Design review of the part built by this model. Coordinates are the model's own, in mm. Coordinates: 2 decimals unless noted, no trailing zeros. Loops run counter-clockwise (first coordinate to the right, second up) from the corner with the lowest first, then second, coordinate; pieces in that order, holes last. Notation, with made-up numbers: (41.5, 57) -> (72.5, 57) arc R22 ccw to (72.5, 93) -> close; hole circle Ø7 at (50.5, 54.5). An arc over 180 degrees is marked (long way). Use one line per item in the form item = value. Start each with the question number.
1. Consider section B-B (z = -2.5). State how many separate pieces and enclosed holes the cut face has, then the cut area to 3 significant figures.
2. Consider section D-D (y = -86). State the section outline as (x, z) points.
3. Consider section C-C (x = 68). State the section outline as (y, z) points, then the cut area to 3 significant figures.
4. For pin 1 (3 mm diameter, centred on x = 131.76, y = 19.05, fed in from +Z); pin 2 (1.5 mm diameter, centred on x = -48, z = -1, fed in from -Y); pin 3 (1.6 mm diameter, centred on x = 122.5, z = -2.5, fed in from -Y), all flat-tipped, find the tip position at first contact; note any pin that passes through.
5. The part is to be moulded in two halves that separate along X. For faces 1 (the face through (-4.716, -75.824, -1.609)), 2 (the face through (-51.9, -11.8, -1.6)), 3 (the face through (35.69, -25.25, -1.65)), say which applies: released by +X, released by -X, zero draft, split by the parting line, or undercut.
6. Consider section A-A (y = -19.05). State the section outline as (x, z) points, then the cut area to 3 significant figures.
7. Wall thickness on line 1 (Y direction, x = 99, z = -1.95); line 2 (X direction, y = -29.5, z = -0.95): over which ranges is each line inside the solid? List them lowest first. Write a range as from..to.
from build123d import *

# Parameters (mm, degrees)
SKETCH1_W                    = 158.75
SKETCH1_H                    = 63.5
BASE_FLANGE1_DEPTH           = 3.2639
F_10_0_1935_DIAMETER_HOLE1_D = 4.9149
BOSS_EXTRUDE1_DEPTH          = 3.2639
F_10_0_1935_DIAMETER_HOLE2_D = 4.9149
FILLET1_R                    = 6.35
FILLET2_R                    = 12.7


# Sheet-metal steps are written as plain solids
with BuildPart() as part:
    # Sketch1 → Base-Flange1 (new body)
    with BuildSketch(Plane.XY):
        with Locations((79.375, 0)):
            Rectangle(SKETCH1_W, SKETCH1_H)
    extrude(amount=-BASE_FLANGE1_DEPTH)

    # #10 (0.1935) Diameter Hole1 (through all)
    with Locations(Plane.XY):
        with Locations((55.5625, 19.05), (55.5625, -19.05), (131.7625, 19.05), (131.7625, -19.05)):
            Hole(F_10_0_1935_DIAMETER_HOLE1_D / 2)

    # Sketch8 → Boss-Extrude1 (add)
    with BuildSketch(Plane.XY):
        Polygon((0, 31.75), (-108.232504257, -59.067854404), (-57.211237738, -119.872632076), (47.809225627, -31.75), (0, -31.75), align=None)
    extrude(amount=-BOSS_EXTRUDE1_DEPTH)

    # #10 (0.1935) Diameter Hole2 (through all)
    with Locations(Plane.XY):
        with Locations((-1.369691562, 16.094353813), (-96.225144731, -63.498821956), (35.365620332, -27.685086111), (-59.489832837, -107.27826188)):
            Hole(F_10_0_1935_DIAMETER_HOLE2_D / 2)

    # Fillet1
    fillet1_edges = [part.edges().sort_by_distance(p)[0] for p in [
        (-108.232504257, -59.067854404, -1.63195),
        (-57.211237738, -119.872632076, -1.63195),
        (0, 31.75, -1.63195),
        (158.75, 31.75, -1.63195),
        (158.75, -31.75, -1.63195),
    ]]
    fillet(fillet1_edges, radius=FILLET1_R)

    # Fillet2
    fillet2_edges = [part.edges().sort_by_distance(p)[0] for p in [
        (47.809225627, -31.75, -1.63195),
    ]]
    fillet(fillet2_edges, radius=FILLET2_R)


solid = part.part
Geometry check:
q1.separate_pieces = 1
q1.enclosed_holes = 8
q1.area = 19,400 mm²
q2.outline = (-85.63, -3.26) -> (-16.84, -3.26) -> (-16.84, 0) -> (-85.63, 0) -> close
q3.outline = (-31.75, -3.26) -> (31.75, -3.26) -> (31.75, 0) -> (-31.75, 0) -> close
q3.area = 207 mm²
q4.pin_1 = through
q4.pin_2 = -112.77
q4.pin_3 = -31.75
q5.face_1 = released by +X
q5.face_2 = released by -X
q5.face_3 = undercut
q6.outline = (-60.54, -3.26) -> (53.11, -3.26) -> (53.11, 0) -> (-60.54, 0) -> close; (58.02, -3.26) -> (129.31, -3.26) -> (129.31, 0) -> (58.02, 0) -> close; (134.22, -3.26) -> (158.75, -3.26) -> (158.75, 0) -> (134.22, 0) -> close
q6.area = 684 mm²
q7.line_1 = -31.75..31.75
q7.line_2 = -72.99..33.71, 37.02..157.25
